CAD build for the part. Positions are in the model's coordinates, mm. Face numbers are marked on the shaded views. Coordinates: 2 decimals unless noted, no trailing zeros. Loops run counter-clockwise (first coordinate to the right, second up) from the corner with the lowest first, then second, coordinate; pieces in that order, holes last. Notation, with made-up numbers: (20, -17) -> (39, -17) arc R24 ccw to (39, -2) -> close; hole circle Ø8 at (46, -25). An arc over 180 degrees is marked (long way). Answer as a JSON object with one key per item and string values. Group by question number.
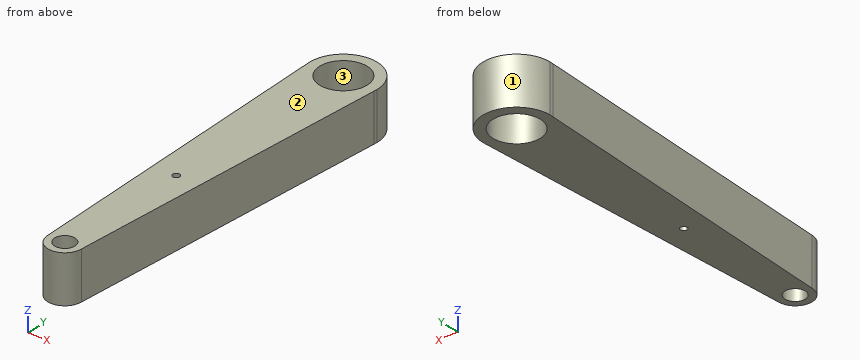
from build123d import *

# Parameters (mm, degrees)
SKETCH1_R           = 1.5
SKETCH1_R_2         = 0.5
SKETCH1_R_3         = 3.5
BOSS_EXTRUDE1_DEPTH = 7
SKETCH1_4_R         = 0.5
BOSS_EXTRUDE2_DEPTH = 5
SKETCH1_5_R         = 0.5
CUT_EXTRUDE3_DEPTH  = 17


with BuildPart() as part:
    # Sketch1 → Boss-Extrude1 (new body)
    with BuildSketch(Plane.XY):
        with BuildLine():
            Line((4.975062344, 29.501246883), (5, 30))
            ThreePointArc((5, 30), (0, 35), (-5, 30))
            Line((-5, 30), (-4.975062344, 29.501246883))
            Line((-4.975062344, 29.501246883), (-2.5, -20))
            ThreePointArc((-2.5, -20), (0, -22.5), (2.5, -20))
            Line((2.5, -20), (4.975062344, 29.501246883))
        make_face()
        with Locations((0, -20)):
            Circle(SKETCH1_R, mode=Mode.SUBTRACT)
        Circle(SKETCH1_R_2, mode=Mode.SUBTRACT)
        with Locations((0, 30)):
            Circle(SKETCH1_R_3, mode=Mode.SUBTRACT)
    extrude(amount=BOSS_EXTRUDE1_DEPTH)

    # Sketch1<4> → Boss-Extrude2 (add)
    with BuildSketch(Plane.XY):
        Circle(SKETCH1_4_R)
    extrude(amount=BOSS_EXTRUDE2_DEPTH)

    # Sketch1<5> → Cut-Extrude3 (cut)
    with BuildSketch(Plane.XY):
        Circle(SKETCH1_5_R)
    extrude(amount=CUT_EXTRUDE3_DEPTH, mode=Mode.SUBTRACT)


solid = part.part
Item 1: Band-saw the part on D-D, the plane y = -19. List the corners of the cut face in (x, z), and give its area (3 significant figures).
Item 2: Band-saw the part on C-C, the plane z = 4. List the corners of the cut face in (x, y).
Item 3: Flat gauge pins, fed straight in: P1, Ø3, axis at y = 21.5, z = 4, coming from the -X side; P2, Ø3, axis at x = -2, y = 25, coming from the -Z side. Where does each tip first touch, or does it go through?
Item 4: Band-saw the part on B-B, the plane y = 0. List the corners of the cut face in (x, z), and give its area (3 significant figures).
Item 5: Pull direction Y, two halves, no side cores. Call the marked faces 1, 2 and 3: +Y half, -Y half, draft (parallel to the pull), parting line (faces both ways), or undercut.
Item 6: Drill centre lines: L1, parallel to Y at x = 0, z = 2; L2, parallel to Y at x = 2, z = 4.5; L3, parallel to X at y = 31.5, z = 6. Where is each one in solid material? Low to high.
Item 7: Band-saw the part on A-A, the plane x = 0. List the corners of the cut face in (y, z).
Reply:
{
 "1": {"outline": "(-2.55, 0) -> (-1.12, 0) -> (-1.12, 7) -> (-2.55, 7) -> close; (1.12, 0) -> (2.55, 0) -> (2.55, 7) -> (1.12, 7) -> close", "area": "20.0 mm²"},
 "2": {"outline": "(-5, 30) -> (-2.5, -20) arc R2.5 ccw to (2.5, -20) -> (5, 30) arc R5 ccw to start; hole circle Ø7 at (0, 30); hole circle Ø3 at (0, -20); hole circle Ø1 at (0, 0)"},
 "3": {"P1": "x = -4.65", "P2": "z = 0"},
 "4": {"outline": "(-3.5, 0) -> (-0.5, 0) -> (-0.5, 7) -> (-3.5, 7) -> close; (0.5, 0) -> (3.5, 0) -> (3.5, 7) -> (0.5, 7) -> close", "area": "42.0 mm²"},
 "5": {"face 1": "+Y half", "face 2": "draft", "face 3": "undercut"},
 "6": {"L1": "-22.5 to -21.5, -18.5 to -0.5, 0.5 to 26.5, 33.5 to 35", "L2": "-21.5 to 27.13, 32.87 to 34.58", "L3": "-4.77 to -3.16, 3.16 to 4.77"},
 "7": {"outline": "(-22.5, 0) -> (-21.5, 0) -> (-21.5, 7) -> (-22.5, 7) -> close; (-18.5, 0) -> (-0.5, 0) -> (-0.5, 7) -> (-18.5, 7) -> close; (0.5, 0) -> (26.5, 0) -> (26.5, 7) -> (0.5, 7) -> close; (33.5, 0) -> (35, 0) -> (35, 7) -> (33.5, 7) -> close"}
}
